Build history of the part. All positions in model axes, mm. A direction names the side the tool comes from. Round coordinates to 2 decimals unless told otherwise and drop trailing zeros. Loops run counter-clockwise (first coordinate to the right, second up) from the corner with the lowest first, then second, coordinate; pieces in that order, holes last. Notation, with made-up numbers: (23, 22) -> (79, 22) arc R18 cw to (79, 53) -> close; hole circle Ø6 at (-26.5, 50). An arc over 180 degrees is marked (long way). Put each result on its own line as item: value. Start each with the question number.
Item 1: Cut at A-A, the plane y = 33. List the corners of the cut face in (x, z), plus the area to 3 significant figures.
Item 2: Tool access for faces 5 (the flat face through (21, 30, -3)), 6 (the cylindrical face through (21, 20, -7)), 7 (the flat face through (12.4, 20.1, -4)), 8 (the flat face through (21, 10, -3)): list every direction of +Z, -Z, +X, -X, +Y, -Y with a clear straight run to the whole face (end or side of a thin tool).
Item 3: Pull direction X, two halves, no side cores. Call faces 1 (the flat face through (5.9, 0, 0.5)), 2 (the cylindrical face through (8.385, 7.251, 0.493)), 3 (the flat face through (12, 33.9, 0.5)), 4 (the cylindrical face through (7.34, 33.61, 0.49)): +X half, -X half, draft (parallel to the pull), parting line (faces both ways), or undercut.
Item 4: Flat gauge pins, fed straight in: pin 1 Ø2 at (y, z) = (30.5, -2) entering from -X; pin 2 Ø12 at (x, y) = (13.5, 5) entering from -Z; pin 3 Ø1.1 at (y, z) = (3.5, 0.5) entering from +X; pin 4 Ø4 at (x, y) = (15.5, 7.5) entering from -Z. Where does each tip first touch, or does it go through?
Item 5: Cut at C-C, the plane x = 19. List the corners of the cut face in (y, z), plus the area to 3 significant figures.
Item 6: Cut at D-D, the plane y = 11.5. List the corners of the cut face in (x, z), plus the area to 3 significant figures.
Item 7: Drill centre lines: probe 1 along Y at (x, z) = (6, 0.65); probe 2 along X at (y, z) = (12.5, -4.25); probe 3 along Z at (x, y) = (17, 27.5). Where is each one in solid material? Low to high. Write a range as [from, to].
Item 8: Cut at B-B, the plane x = 6. List the corners of the cut face in (y, z).
```python
from build123d import *

# Parameters (mm, degrees)
SKETCH_1_W      = 12
SKETCH_1_H      = 38
SKETCH_1_R      = 2.5
EXTRUDE_1_DEPTH = 1
EXTRUDE_2_DEPTH = 20


with BuildPart() as part:
    # 草图1 → 凸台-拉伸1 (new body)
    with BuildSketch(Plane.XY):
        with Locations((6, 19)):
            Rectangle(SKETCH_1_W, SKETCH_1_H)
        with Locations((6, 31.5)):
            Circle(SKETCH_1_R, mode=Mode.SUBTRACT)
        with Locations((6, 6.5)):
            Circle(SKETCH_1_R, mode=Mode.SUBTRACT)
    extrude(amount=EXTRUDE_1_DEPTH)

    # 草图2 → 凸台-拉伸2 (add)
    with BuildSketch(Plane(origin=(0, 30, 0), x_dir=(1, 0, 0), z_dir=(0, 1, 0))):
        with BuildLine():
            Line((12, 0), (12, -1))
            Line((12, -1), (17, -1))
            ThreePointArc((17, -1), (20.535533906, 7.535533906), (12, 4))
            Line((12, 4), (12.902768587, 4))
            ThreePointArc((12.902768587, 4), (19.731195711, 6.828427125), (16.902768587, 0))
            Line((16.902768587, 0), (12, 0))
        make_face()
    extrude(amount=-EXTRUDE_2_DEPTH)


solid = part.part
```
Reply:
1. outline: (0, 0) -> (4, 0) -> (4, 1) -> (0, 1) -> close; (8, 0) -> (12, 0) -> (12, 1) -> (8, 1) -> close
1. area: 8.00 mm^2
2. face 5: +Z, -Z, +X, +Y
2. face 6: +Y, -Y
2. face 7: -X, +Y, -Y
2. face 8: +Z, -Z, +X, -Y
3. face 1: draft
3. face 2: undercut
3. face 3: +X half
3. face 4: undercut
4. pin 1: stops at x = 19.69
4. pin 2: stops at z = -9
4. pin 3: stops at x = 12
4. pin 4: passes through
5. outline: (10, -8.58) -> (30, -8.58) -> (30, -7.41) -> (10, -7.41) -> close; (10, -0.59) -> (30, -0.59) -> (30, 0.58) -> (10, 0.58) -> close
5. area: 47.1 mm^2
6. outline: (0, 0) -> (16.9, 0) arc R4 cw (long way) to (12.9, -4) -> (12, -4) arc R5 ccw (long way) to (17, 1) -> (0, 1) -> close
6. area: 38.6 mm^2
7. probe 1: y = [0, 4], [9, 29], [34, 38]
7. probe 2: x = [12.01, 12.91], [20.89, 21.99]
7. probe 3: z = [-9, -8], [0, 1]
8. outline: (0, 0) -> (4, 0) -> (4, 1) -> (0, 1) -> close; (9, 0) -> (29, 0) -> (29, 1) -> (9, 1) -> close; (34, 0) -> (38, 0) -> (38, 1) -> (34, 1) -> close
